Geometry check sheet. Reference: drawing and pictorial views, mm from the part's lowest x, y, z. A direction names the side the tool comes from. Give positions to 0.01 mm unless a question says otherwise; leave off trailing zeros. Write each loop counter-clockwise with the first axis right and the second up, starting at its lowest first coordinate (ties: lowest second). Pieces come first, ordered by that corner, then holes. Notation, with made-up numbers: (2.25, 65) - (53.25, 65) arc R30 cw to (53.25, 93) - close; hole circle Ø7 at (39, 41.25). An arc over 180 degrees is marked (long way). Put each result on its own line as item: value.
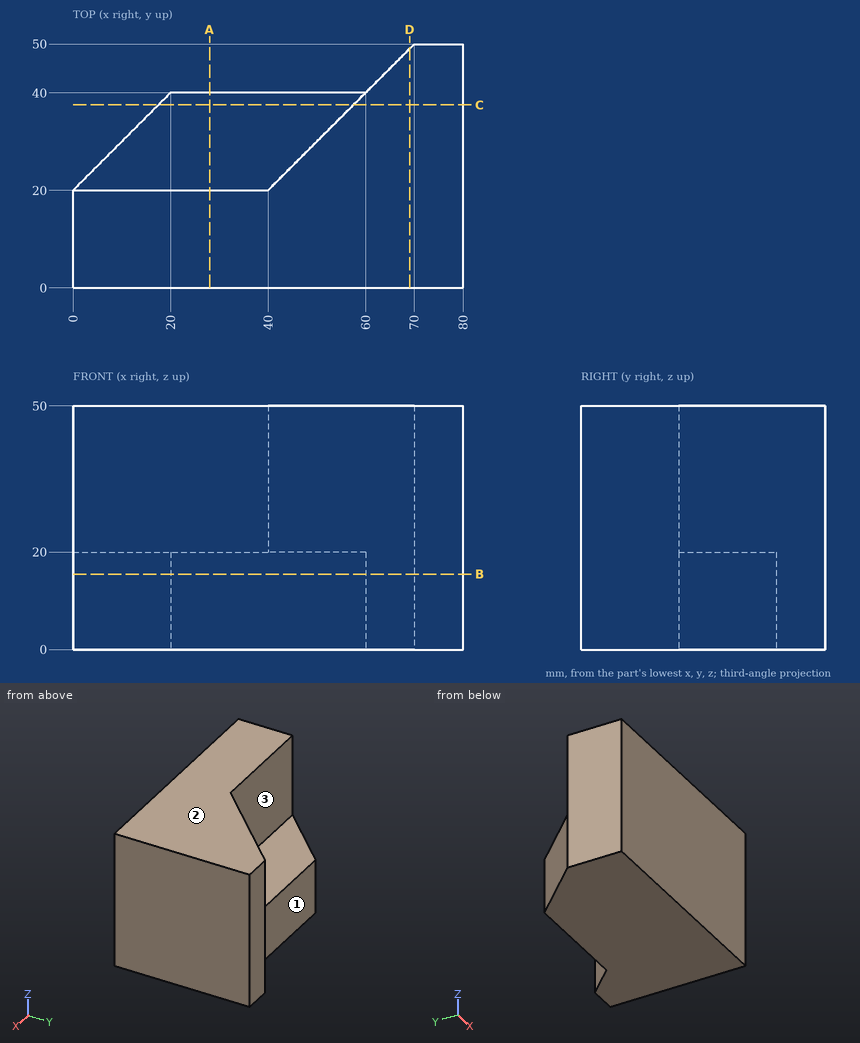
Q1. Section check A-A, the plane x = 28. Record the cut outline in (y, z), plus the area to 3 significant figures.
Answers follow:
outline: (0, 0) - (40, 0) - (40, 20) - (20, 20) - (20, 50) - (0, 50) - close
area: 1,400 mm2
Q2. Set-up check for the marked faces 1, 2 and 3: record each of +Z, -Z, +X, -X, +Y, -Y from which the full face is reachable in a straight line by a thin tool's end or side.
Answers follow:
face 1: +Z, -Z, -X, +Y
face 2: +Z, +X, -X, +Y, -Y
face 3: +Z, -X, +Y
Q3. Go/stop test with flat-tipped pins: pin 1 Ø12 at (y, z) = (38.5, 18) entering from -X; pin 2 Ø6 at (x, z) = (35.5, 7) entering from +Y; pin 3 Ø15 at (x, z) = (23.5, 33) entering from +Y. Record where each tip stops, or that it passes through.
Answers follow:
pin 1: stops at x = 12.5
pin 2: stops at y = 40
pin 3: stops at y = 20
Q4. Section check C-C, the plane y = 37.5. Record the cut outline in (x, z).
Answers follow:
outline: (17.5, 0) - (80, 0) - (80, 50) - (57.5, 50) - (57.5, 20) - (17.5, 20) - close
Q5. Scan lines: line 1 along Z through (x, y) = (52, 36.5); line 2 along Y through (x, z) = (26, 16). Record each from-to range of solid material in increasing order.
Answers follow:
line 1: z = 0 to 20
line 2: y = 0 to 40
Q6. Section check D-D, the plane x = 69. Record the cut outline in (y, z), plus the area to 3 significant figures.
Answers follow:
outline: (0, 0) - (49, 0) - (49, 50) - (0, 50) - close
area: 2,450 mm2
Q7. Section check B-B, the plane z = 15.5. Record the cut outline in (x, y), plus the area to 3 significant figures.
Answers follow:
outline: (0, 0) - (80, 0) - (80, 50) - (70, 50) - (60, 40) - (20, 40) - (0, 20) - close
area: 3,150 mm2
